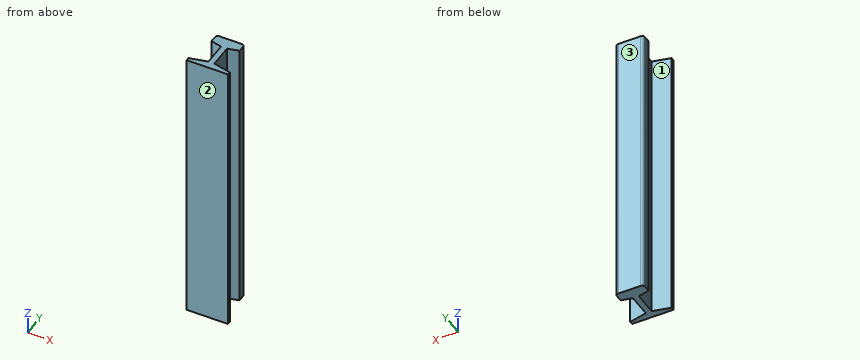
Autodesk Inventor part; units mm, degrees
ref_plane "YZ Plane" through (0, 0, 0) normal (1, 0, 0) x (0, 1, 0)
ref_plane "XZ Plane" through (0, 0, 0) normal (0, 1, 0) x (-1, 0, 0)
ref_plane "XY Plane" through (0, 0, 0) normal (0, 0, 1) x (1, 0, 0)
sketch "Sketch1" plane through (0, 0, 0) normal (0, 0, 1) x (1, 0, 0)
  line L0 (0, 0) -> (3.7042, 0)
  line L1 (1.8521, 0) -> (1.8521, 0.6615)
  line L2 (1.8521, 0.6615) -> (2.1167, 0.6615)
  line L3 (2.1167, 0.6615) -> (3.7042, 0.295)
  line L4 (3.7042, 0.295) -> (3.7042, 0)
  line L5 (1.8521, 0.6615) -> (1.8521, 2.7781)
  line L6 (1.8521, 2.7781) -> (2.1167, 2.7781)
  line L7 (2.1167, 2.7781) -> (2.1167, 0.6615)
  line L8 (1.8521, 2.7781) -> (1.8521, 3.8365)
  line L9 (1.8521, 3.8365) -> (2.8549, 3.8365)
  line L10 (2.1167, 2.7781) -> (3.1089, 3.0072)
  line L11 (2.1167, 2.7781) -> (3.135, 2.7781) construction
  line L12 (3.1089, 3.5825) -> (3.1089, 3.0072)
  arc A0 (3.1089, 3.5825) -> (2.8549, 3.8365) centre (2.8549, 3.5825) ccw
  line L13 (3.7042, 0) -> (0, 0)
  line L14 (1.8521, 0.6615) -> (1.5875, 0.6615)
  line L15 (1.5875, 0.6615) -> (0, 0.295)
  line L16 (0, 0.295) -> (0, 0)
  line L17 (1.8521, 2.7781) -> (1.5875, 2.7781)
  line L18 (1.5875, 2.7781) -> (1.5875, 0.6615)
  line L19 (1.8521, 3.8365) -> (0.8493, 3.8365)
  line L20 (1.5875, 2.7781) -> (0.5953, 3.0072)
  line L21 (1.5875, 2.7781) -> (0.5692, 2.7781) construction
  line L22 (0.5953, 3.5825) -> (0.5953, 3.0072)
  arc A1 (0.8493, 3.8365) -> (0.5953, 3.5825) centre (0.8493, 3.5825) ccw
  dimension "d3" = 0.6615
  dimension "d4" = 0.2646
  dimension "d5" = 167
  dimension "d6" = 2.1167
  dimension "d7" = 1.0583
  dimension "d9" = 13
  dimension "d10" = 0.254
extrude "Extrusion1" add sketch "Sketch1" against normal blind 25.4
properties part number "Rail48in"
Read the model definition and answer for the solid it produces. Units are mm, in the model's axes. Face numbers are marked on the shaded views. Coordinates: 2 decimals unless noted, no trailing zeros. Order: outer loops, then holes, each group sorted by start corner. A loop starts at its lowest first (then second) coordinate and runs counter-clockwise, first axis right, second up. Notation, with made-up numbers: (30.25, -22.5) - (37.25, -22.5) arc R19 ccw to (37.25, -15.5) - close; hole circle Ø2 at (51, -26.75). An arc over 180 degrees is marked (long way). Answer as a JSON object with one key per item and string values. Group by question number.
Item 1: Section B-B (x = 2.5) is taken. Give the vertices of the cut face in (y, z).
Item 2: Consider probe 1 along X at (y, z) = (1, -3.5); probe 2 along Y at (x, z) = (1, -13.25); probe 3 along Y at (x, z) = (1.2, -5.5). Determine where each line is inside the solid, lowest interval first. Write a range as from..to.
Item 3: Section C-C (y = 1.2) is taken. Give the vertices of the cut face in (x, z), plus the area to 3 significant figures.
Item 4: The mould has two halves that part along Y. Classify the marked faces 1, 2 and 3: +Y half, -Y half, draft (parallel to the pull), parting line (faces both ways), or undercut.
Item 5: Flat-ended cylindrical pins translate along their axes: P1, Ø0.6, axis at y = 3.5, z = -12.5, coming from the +X side; P2, Ø0.6, axis at y = 2, z = -16.5, coming from the +X side; P3, Ø1, axis at x = 0.5, y = 2, coming from the -Z side (3 decimals). Find the tip coordinate at first contact, or state that the pin passes through.
Results are:
{
 "1": {"outline": "(0, -25.4) - (0.57, -25.4) - (0.57, 0) - (0, 0) - close; (2.87, -25.4) - (3.84, -25.4) - (3.84, 0) - (2.87, 0) - close"},
 "2": {"probe 1": "x = 1.59..2.12", "probe 2": "y = 0..0.53, 2.91..3.84", "probe 3": "y = 0..0.57, 2.87..3.84"},
 "3": {"outline": "(1.59, -25.4) - (2.12, -25.4) - (2.12, 0) - (1.59, 0) - close", "area": "13.4 mm^2"},
 "4": {"face 1": "undercut", "face 2": "-Y half", "face 3": "+Y half"},
 "5": {"P1": "stops at x = 3.11", "P2": "stops at x = 2.12", "P3": "passes through"}
}
